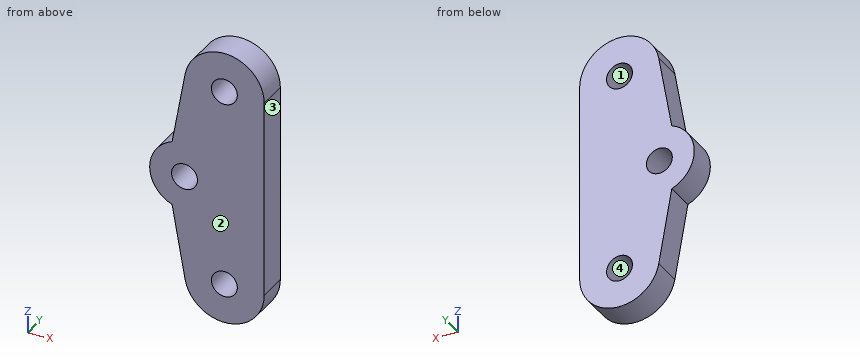
Autodesk Fusion 360 part; units mm, degrees
sketch "Sketch1" plane through (0, 0, 0) normal (0, 1, 0) x (1, 0, 0)
  line L0 (0, 0) -> (0, -20) construction
  circle A0 centre (0, 0) radius 2.6
  circle A1 centre (8, -20) radius 2.6
  line L1 (0, -20) -> (8, -20) construction
  line L2 (0, 0) -> (18.1281, 0) construction
  circle A2 centre (8, 20) radius 2.6
  circle A3 centre (8, 20) radius 8
  circle A4 centre (0, 0) radius 7
  circle A5 centre (8, -20) radius 8
  line L3 (16, 20) -> (16, -20)
  line L4 (0.4465, 22.6352) -> (0.4465, 23.2319)
  line L5 (0.4465, 23.2319) -> (-2.4969, 6.5396)
  line L6 (0.4465, -23.2319) -> (-2.4969, -6.5396)
  dimension "d1" = 5.2
  dimension "d2" = 8
  dimension "d3" = 20
  dimension "d4" = 16
  dimension "d5" = 14
  dimension "d8" = 10
extrude "Extrude1" add sketch "Sketch1" along normal blind 6 contours A3 | A3 A4 A5 L3 L5 L6 | A5 | A4
The listing builds one solid part. Answer for the finished solid, in the listing's coordinates (mm). Face numbers are marked on the shaded views. Coordinates: 2 decimals unless noted, no trailing zeros. Order: outer loops, then holes, each group sorted by start corner. A loop starts at its lowest first (then second) coordinate and runs counter-clockwise, first axis right, second up. Notation, with made-up numbers: (42, 50) -> (81, 50) arc R17 ccw to (81, 58) -> close; hole circle Ø9 at (85.25, 61.25). An arc over 180 degrees is marked (long way). Answer in a Markdown table with one row per item. Add a question column.
Item 1: Find section C-C (y = 0.65). Write down the section's boundary in (x, z).
Item 2: Find section B-B (z = 0). Write down the section's boundary in (x, y), then the cut area to 3 significant figures.
Item 3: Determine the mould class of the marked faces 1, 2, 3 and 4 for opening direction X: +X half, -X half, draft (parallel to the pull), parting line (faces both ways), or undercut.
Item 4: Find the intervals of material crossed by L1, parallel to Z at x = 8, y = 2.15; L2, parallel to X at y = 2.25, z = 0; L3, parallel to Z at x = 9.5, y = 5.55, in increasing order. Write a range as from..to.
Item 5: Find section A-A (x = 8). Write down the section's boundary in (y, z).
Item 6: Find section D-D (z = -22). Write down the section's boundary in (x, y), then the cut area to 3 significant figures.
Result set:
| question | item | result |
|---|---|---|
| 1 | outline | (-2.5, -6.54) -> (0.12, -21.39) arc R8 ccw to (16, -20) -> (16, 20) arc R8 ccw to (0.12, 21.39) -> (-2.5, 6.54) arc R7 ccw to start; hole circle Ø5.2 at (0, 0); hole circle Ø5.2 at (8, -20); hole circle Ø5.2 at (8, 20) |
| 2 | outline | (-7, 0) -> (-2.6, 0) -> (-2.6, 6) -> (-7, 6) -> close; (2.6, 0) -> (16, 0) -> (16, 6) -> (2.6, 6) -> close |
| 2 | area | 107 mm² |
| 3 | face 1 | undercut |
| 3 | face 2 | draft |
| 3 | face 3 | +X half |
| 3 | face 4 | undercut |
| 4 | L1 | z = -28..-22.6, -17.4..17.4, 22.6..28 |
| 4 | L2 | x = -7..-2.6, 2.6..16 |
| 4 | L3 | z = -27.86..-22.12, -17.88..17.88, 22.12..27.86 |
| 5 | outline | (0, -28) -> (6, -28) -> (6, -22.6) -> (0, -22.6) -> close; (0, -17.4) -> (6, -17.4) -> (6, 17.4) -> (0, 17.4) -> close; (0, 22.6) -> (6, 22.6) -> (6, 28) -> (0, 28) -> close |
| 6 | outline | (0.25, 0) -> (6.34, 0) -> (6.34, 6) -> (0.25, 6) -> close; (9.66, 0) -> (15.75, 0) -> (15.75, 6) -> (9.66, 6) -> close |
| 6 | area | 73.0 mm² |
